```python
from build123d import *

# Parameters (mm, degrees)
F1_DEPTH  = 17
F2_DEPTH  = 5
F3_DEPTH  = 17
F4_DEPTH  = 3
F5_W      = 17.619991675
F5_H      = 2.2976936506
F6_DEPTH  = 10
F7_W      = 10
F7_H      = 4
F7_W_2    = 40
F7_H_2    = 5
F8_DEPTH  = 3
F9_W      = 6
F9_H      = 6
F10_DEPTH = 3


# Not quite as in the source:
# - a feature names something its author has since deleted; it is built from what else it names


with BuildPart() as f1:
    # F0 (on Top) → F1 (new body)
    with BuildSketch(Plane.XY):
        with BuildLine():
            Line((24.3022678875, 34), (-24.3022678875, 34))
            ThreePointArc((-24.3022678875, 34), (-29.745386464, 31.745386464), (-32, 26.3022678875))
            Line((-32, 26.3022678875), (-32, 15.1276998222))
            Line((-32, 15.1276998222), (-30.5, 15.1276998222))
            Line((-30.5, 15.1276998222), (-30.5, 21.3020170704))
            Line((-30.5, 21.3020170704), (30.5, 21.3020170704))
            Line((30.5, 21.3020170704), (30.5, 14.2477769405))
            Line((30.5, 14.2477769405), (32, 14.2477769405))
            Line((32, 14.2477769405), (32, 26.3022678875))
            ThreePointArc((32, 26.3022678875), (29.745386464, 31.745386464), (24.3022678875, 34))
        make_face()
        with BuildLine():
            Line((-30.5, 15.1276998222), (-32, 15.1276998222))
            Line((-32, 15.1276998222), (-32, -26.3022678875))
            ThreePointArc((-32, -26.3022678875), (-29.745386464, -31.745386464), (-24.3022678875, -34))
            Line((-24.3022678875, -34), (0, -34))
            Line((0, -34), (0, -32))
            Line((0, -32), (-20, -32))
            Line((-20, -32), (-20, -27.4899639189))
            Line((-20, -27.4899639189), (-20.3994758379, -27.4899639189))
            ThreePointArc((-20.3994758379, -27.4899639189), (-30.2031719041, -25.7844938681), (-20.255592559, -25.5261339915))
            Line((-20.255592559, -25.5261339915), (-20, -25.5261339915))
            Line((-20, -25.5261339915), (-20, -22.0704134554))
            Line((-20, -22.0704134554), (-4.1499226354, -22.0704134554))
            Line((-4.1499226354, -22.0704134554), (-4.1499226354, -14.6979829296))
            Line((-4.1499226354, -14.6979829296), (-30.5, -14.6979829296))
            Line((-30.5, -14.6979829296), (-30.5, 15.1276998222))
        make_face()
        with BuildLine():
            Line((32, -26.3022678875), (32, 14.2477769405))
            Line((32, 14.2477769405), (30.5, 14.2477769405))
            Line((30.5, 14.2477769405), (30.5, -14.6979829296))
            Line((30.5, -14.6979829296), (4.1499226354, -14.6979829296))
            Line((4.1499226354, -14.6979829296), (4.1499226354, -22.0704134554))
            Line((4.1499226354, -22.0704134554), (20, -22.0704134554))
            Line((20, -22.0704134554), (20, -25.4029799253))
            Line((20, -25.4029799253), (20.2726339823, -25.4029799253))
            ThreePointArc((20.2726339823, -25.4029799253), (25.5910239568, -21.1638916046), (30.2165381279, -26.1498479185))
            ThreePointArc((30.2165381279, -26.1498479185), (25.7296627026, -31.1234485429), (20.3218568596, -27.1706786007))
            Line((20.3218568596, -27.1706786007), (20, -27.1706786007))
            Line((20, -27.1706786007), (20, -32))
            Line((20, -32), (0, -32))
            Line((0, -32), (0, -34))
            Line((0, -34), (24.3022678875, -34))
            ThreePointArc((24.3022678875, -34), (27.9138443036, -33.100178998), (30.6810753302, -30.6110838832))
            ThreePointArc((30.6810753302, -30.6110838832), (31.6628871063, -28.555346757), (32, -26.3022678875))
        make_face()
        Polygon((-30.5, 21.3020170704), (-30.5, 15.1276998222), (-30.5, -14.6979829296), (-4.1499226354, -14.6979829296), (4.1499226354, -14.6979829296), (30.5, -14.6979829296), (30.5, 14.2477769405), (30.5, 21.3020170704), align=None)
        Polygon((4.1499226354, -14.6979829296), (-4.1499226354, -14.6979829296), (-4.1499226354, -22.0704134554), (0, -22.0704134554), (4.1499226354, -22.0704134554), align=None)
        with BuildLine():
            ThreePointArc((20.2726339823, -25.4029799253), (20.2184754644, -26.2890226707), (20.3218568596, -27.1706786007))
            ThreePointArc((20.3218568596, -27.1706786007), (25.7296627026, -31.1234485429), (30.2165381279, -26.1498479185))
            ThreePointArc((30.2165381279, -26.1498479185), (25.5910239568, -21.1638916046), (20.2726339823, -25.4029799253))
        make_face()
    extrude(amount=F1_DEPTH)

    # F0 (on Top) → F2 (cut)
    with BuildSketch(Plane.XY):
        Polygon((-30.5, 21.3020170704), (-30.5, 15.1276998222), (-30.5, -14.6979829296), (-4.1499226354, -14.6979829296), (4.1499226354, -14.6979829296), (30.5, -14.6979829296), (30.5, 14.2477769405), (30.5, 21.3020170704), align=None)
        Polygon((4.1499226354, -14.6979829296), (-4.1499226354, -14.6979829296), (-4.1499226354, -22.0704134554), (0, -22.0704134554), (4.1499226354, -22.0704134554), align=None)
    extrude(amount=F2_DEPTH, mode=Mode.SUBTRACT)

    # F0 (on Top) → F3 (join)
    with BuildSketch(Plane.XY):
        with BuildLine():
            ThreePointArc((-20.255592559, -25.5261339915), (-30.2031719041, -25.7844938681), (-20.3994758379, -27.4899639189))
            ThreePointArc((-20.3994758379, -27.4899639189), (-20.2624836545, -26.8261202565), (-20.2165381279, -26.1498479185))
            ThreePointArc((-20.2165381279, -26.1498479185), (-20.2263112871, -25.8373801956), (-20.255592559, -25.5261339915))
        make_face()
    extrude(amount=F3_DEPTH)

    # F0 (on Top) → F4 (cut)
    with BuildSketch(Plane.XY):
        with BuildLine():
            ThreePointArc((20.2726339823, -25.4029799253), (20.2184754644, -26.2890226707), (20.3218568596, -27.1706786007))
            ThreePointArc((20.3218568596, -27.1706786007), (25.7296627026, -31.1234485429), (30.2165381279, -26.1498479185))
            ThreePointArc((30.2165381279, -26.1498479185), (25.5910239568, -21.1638916046), (20.2726339823, -25.4029799253))
        make_face()
        with BuildLine():
            ThreePointArc((-20.255592559, -25.5261339915), (-30.2031719041, -25.7844938681), (-20.3994758379, -27.4899639189))
            ThreePointArc((-20.3994758379, -27.4899639189), (-20.2624836545, -26.8261202565), (-20.2165381279, -26.1498479185))
            ThreePointArc((-20.2165381279, -26.1498479185), (-20.2263112871, -25.8373801956), (-20.255592559, -25.5261339915))
        make_face()
    extrude(amount=F4_DEPTH, mode=Mode.SUBTRACT)

    # F5 (on face) → F6 (cut)
    with BuildSketch(Plane.XY.offset(17)):
        with BuildLine():
            Line((21.7456496224, 31.2272801952), (-21.5543503776, 31.2272801952))
            ThreePointArc((-21.5543503776, 31.2272801952), (-26.0444784382, 29.3674082557), (-27.9043503776, 24.8772801952))
            Line((-27.9043503776, 24.8772801952), (-27.9043503776, -13.4227198048))
            ThreePointArc((-27.9043503776, -13.4227198048), (-26.0444784382, -17.9128478653), (-21.5543503776, -19.7727198048))
            Line((-21.5543503776, -19.7727198048), (-8.8099958375, -19.7727198048))
            Line((-8.8099958375, -19.7727198048), (8.8099958375, -19.7727198048))
            Line((8.8099958375, -19.7727198048), (21.7456496224, -19.7727198048))
            ThreePointArc((21.7456496224, -19.7727198048), (26.2357776829, -17.9128478653), (28.0956496224, -13.4227198048))
            Line((28.0956496224, -13.4227198048), (28.0956496224, 24.8772801952))
            ThreePointArc((28.0956496224, 24.8772801952), (26.2357776829, 29.3674082557), (21.7456496224, 31.2272801952))
        make_face()
        with Locations((0, -20.9215666301)):
            Rectangle(F5_W, F5_H)
    extrude(amount=-F6_DEPTH, mode=Mode.SUBTRACT)

    # F7 (on face) → F8 (cut)
    with BuildSketch(Plane.XY):
        with Locations((-14.1091264039, -18.375430584)):
            Rectangle(F7_W, F7_H)
        with Locations((14.1091264039, -18.375430584)):
            Rectangle(F7_W, F7_H)
        with Locations((-1.1501409858, 27.3545110226)):
            Rectangle(F7_W_2, F7_H_2)
    extrude(amount=F8_DEPTH, mode=Mode.SUBTRACT)

    # F9 (on face) → F10 (cut)
    with BuildSketch(Plane.XY.offset(17)):
        with Locations((25.4528271034, -26.7212770808)):
            Rectangle(F9_W, F9_H)
        with Locations((-25.4528271034, -26.7212770808)):
            Rectangle(F9_W, F9_H)
    extrude(amount=-F10_DEPTH, mode=Mode.SUBTRACT)


solid = f1.part
```
Input: part model. Units: mm. Frame: model coordinates. A direction names the side the tool comes from. Round coordinates to 2 decimals unless told otherwise and drop trailing zeros. Loops run counter-clockwise (first coordinate to the right, second up) from the corner with the lowest first, then second, coordinate; pieces in that order, holes last. Notation, with made-up numbers: (-2, 79) -> (20, 79) arc R25 ccw to (20, 113) -> close; hole circle Ø11 at (55.25, -23). An arc over 180 degrees is marked (long way). One line per item, written item: value.
(1) Section C-C (y = -28.5). Return the cut outline in (x, z).
Geometry check:
outline: (-31.68, 0) -> (-29.63, 0) -> (-29.63, 3) -> (-20.8, 3) -> (-20.8, 0) -> (-20, 0) -> (-20, 17) -> (-22.45, 17) -> (-22.45, 14) -> (-28.45, 14) -> (-28.45, 17) -> (-31.68, 17) -> close; (20, 0) -> (20.8, 0) -> (20.8, 3) -> (29.63, 3) -> (29.63, 0) -> (31.68, 0) -> (31.68, 17) -> (28.45, 17) -> (28.45, 14) -> (22.45, 14) -> (22.45, 17) -> (20, 17) -> close
(2) Section B-B (y = 5). Return the cut outline in (x, z).
Geometry check:
outline: (-32, 0) -> (-30.5, 0) -> (-30.5, 5) -> (30.5, 5) -> (30.5, 0) -> (32, 0) -> (32, 17) -> (28.1, 17) -> (28.1, 7) -> (-27.9, 7) -> (-27.9, 17) -> (-32, 17) -> close
(3) Mould query, pull axis Y, two halves, no side actions, for faces 1 (the face through (-25, -26, 3)), 2 (the face through (0, 34, 8)), 3 (the face through (-22.453, -27, 16)). Classes: pulls with the +Y half, pulls with the -Y half, needs draft (parallel to the pull), parting line crosses it, or undercut.
Geometry check:
face 1: undercut
face 2: pulls with the +Y half
face 3: undercut
(4) Set-up query: faces 4 (the face through (20, -30, 8)), 5 (the face through (-1, 27, 3)), 6 (the face through (-25, -27, 14)). Return all of +Z, -Z, +X, -X, +Y, -Y with unobstructed straight access to the full face (end or side cutting, diameter ignored); none if empty.
Geometry check:
face 4: +Z, -Z
face 5: -Z
face 6: +Z
(5) Material intervals for line 1 (Y direction, x = 0.5, z = 2); line 2 (Y direction, x = -15, z = 1.5); line 3 (Y direction, x = -5, z = 11), sorted ascending. Write a range as [from, to].
Geometry check:
line 1: [-34, -32], [21.3, 24.85], [29.85, 34]
line 2: [-34, -32], [-22.07, -20.38], [-16.38, -14.7], [21.3, 24.85], [29.85, 34]
line 3: [-34, -32], [31.23, 34]
(6) Pin query (flat end, axial travel): pin 1 (2 mm diameter, centred on x = -15.5, y = -4, fed in from -Z); pin 2 (1.5 mm diameter, centred on y = -28, z = 15, fed in from -X). Return the tip coordinate at first contact, or that it passes through.
Geometry check:
pin 1: z = 5
pin 2: x = -31.94
(7) Section D-D (x = -2.5). Return the cut outline in (y, z).
Geometry check:
outline: (-34, 0) -> (-32, 0) -> (-32, 17) -> (-34, 17) -> close; (-22.07, 5) -> (21.3, 5) -> (21.3, 0) -> (24.85, 0) -> (24.85, 3) -> (29.85, 3) -> (29.85, 0) -> (34, 0) -> (34, 17) -> (31.23, 17) -> (31.23, 7) -> (-22.07, 7) -> close
(8) Section A-A (x = -18). Return the cut outline in (y, z).
Geometry check:
outline: (-34, 0) -> (-32, 0) -> (-32, 17) -> (-34, 17) -> close; (-22.07, 0) -> (-20.38, 0) -> (-20.38, 3) -> (-16.38, 3) -> (-16.38, 0) -> (-14.7, 0) -> (-14.7, 5) -> (21.3, 5) -> (21.3, 0) -> (24.85, 0) -> (24.85, 3) -> (29.85, 3) -> (29.85, 0) -> (34, 0) -> (34, 17) -> (31.23, 17) -> (31.23, 7) -> (-19.77, 7) -> (-19.77, 17) -> (-22.07, 17) -> close
